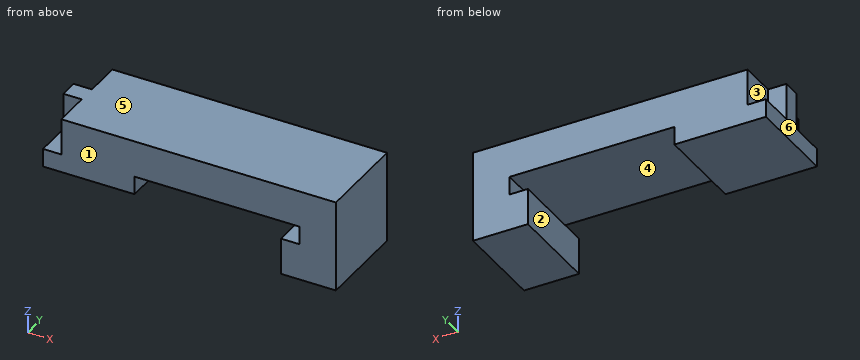
from build123d import *

# Parameters (mm, degrees)
F1_DEPTH = 25
F2_W     = 10
F2_H     = 10
F3_DEPTH = 20


with BuildPart() as f1:
    # F0 (on Front) → F1 (new body, symmetric)
    with BuildSketch(Plane.XZ):
        Polygon((0, 20), (0, 0), (30, 0), (30, 50), (-120, 50), (-120, 30), (-130, 30), (-130, 20), (-80, 20), (-80, 30), (10, 30), (10, 20), align=None)
    extrude(amount=F1_DEPTH, both=True)

    # F2 (on face) → F3 (join, through all)
    with BuildSketch(Plane.XY.offset(30)):
        with Locations((-125, 0)):
            Rectangle(F2_W, F2_H)
    extrude(amount=F3_DEPTH)


solid = f1.part
Design review of the part built by this model. Coordinates are the model's own, in mm. Face numbers are marked on the shaded views. A direction names the side the tool comes from. Round coordinates to 2 decimals unless told otherwise and drop trailing zeros. Loops run counter-clockwise (first coordinate to the right, second up) from the corner with the lowest first, then second, coordinate; pieces in that order, holes last. Notation, with made-up numbers: (-31, 36.25) - (-23, 36.25) arc R19 cw to (-23, 42.25) - close; hole circle Ø6 at (40.5, 7.25). An arc over 180 degrees is marked (long way). One line per item, written item: value. Start each with the question number.
1) Consider section C-C on z = 47.5. Give the boundary of the cut face in (x, y).
2) Draft analysis for pull direction X (two halves, no side actions). For the marked faces 4, 5 and 6, state which applies: +X half, -X half, draft (parallel to the pull), parting line (faces both ways), or undercut.
3) Consider section D-D on x = -114. Give the boundary of the cut face in (y, z).
4) Consider section A-A on z = 25.5. Give the boundary of the cut face in (x, y).
5) Consider section B-B on y = -1. Give the boundary of the cut face in (x, z).
6) Insertion check: pin 1 Ø10 at (y, z) = (16, 45) entering from -X; pin 2 Ø2 at (y, z) = (4, 18) entering from -X; pin 3 Ø5 at (x, z) = (-125, 39.5) entering from -Y. Each pin has a flat end and moves straight along its axis. Give the tip position at first contact, or say it passes through.
7) For the marked faces 1, 2 and 3, list the 3-axis set-ups (+Z, -Z, +X, -X, +Y, -Y) from which the entire face can be reached by the end or side of a thin tool; tool diameter is ignored.
8) To check wall thickness, follow L1, parallel to Z at x = 1.5, y = 0.5; L2, parallel to X at y = 3.5, z = 24; L3, parallel to X at y = -10, z = 41. State the ranges of each line that lie inside material, in increasing order. Write a range as from..to.
Reported:
1. outline: (-130, -5) - (-120, -5) - (-120, -25) - (30, -25) - (30, 25) - (-120, 25) - (-120, 5) - (-130, 5) - close
2. face 4: undercut
2. face 5: draft
2. face 6: -X half
3. outline: (-25, 20) - (25, 20) - (25, 50) - (-25, 50) - close
4. outline: (-130, -25) - (-80, -25) - (-80, 25) - (-130, 25) - close; (10, -25) - (30, -25) - (30, 25) - (10, 25) - close
5. outline: (-130, 20) - (-80, 20) - (-80, 30) - (10, 30) - (10, 20) - (0, 20) - (0, 0) - (30, 0) - (30, 50) - (-130, 50) - close
6. pin 1: stops at x = -120
6. pin 2: stops at x = 0
6. pin 3: stops at y = -5
7. face 1: +Z, -Z, +X, -X, -Y
7. face 2: -Z, -X, +Y, -Y
7. face 3: +Z, -X, +Y
8. L1: z = 0..20, 30..50
8. L2: x = -130..-80, 10..30
8. L3: x = -120..30
